CAD build for the part. Positions are in the model's coordinates, mm. A direction names the side the tool comes from. Round coordinates to 2 decimals unless told otherwise and drop trailing zeros. Order: outer loops, then holes, each group sorted by start corner. A loop starts at its lowest first (then second) coordinate and runs counter-clockwise, first axis right, second up. Notation, with made-up numbers: (69.5, 16) -> (109.5, 16) arc R7 cw to (109.5, 27) -> close; hole circle Ø10 at (-32, -38.75). An arc over 180 degrees is marked (long way). Return JSON: item names as keys, results as strings. Group by question number.
Q1. Cut at B-B (y = 12.25). Write the cut outline in (x, z), then the cut area to 3 significant figures.
Q2. Mould opens along X. For faces 1 (the flat face through (-12, 6, -11.3)), 2 (the cylindrical face through (18.521, 6.374, -3.794)), 3 (the flat face through (-20, 11, 0)) say: +X half, -X half, draft (parallel to the pull), parting line (faces both ways), or undercut.
Q3. Cut at C-C (z = -0.75). Write the cut outline in (x, y).
Q4. Probe line 1 along X through (y, z) = (7.75, -10.75); line 2 along X through (y, z) = (8.75, 9.5); line 3 along Z through (x, y) = (-10.5, 12.5). List the from-to ranges inside material, lowest first.
Q5. Flat gauge pins, fed straight in: pin 1 (2 mm diameter, centred on x = -12, z = -10.5, fed in from +Y); pin 2 (1.6 mm diameter, centred on x = -11.5, y = 6.5, fed in from -Z). Where does each tip first touch, or does it go through?
Q6. Cut at D-D (z = 2.5). Write the cut outline in (x, y), then the cut area to 3 significant figures.
Q7. Cut at A-A (x = 12.5). Write the cut outline in (y, z).
Q8. Which spindle directions (+Z, -Z, +X, -X, +Y, -Y) get a long thin tool onto all of the face, cutting with end or side? Do faces 4 (the flat face through (0, 8.5, 11)), 5 (the flat face through (19, 10, 2)), 6 (the flat face through (-17, 10, 0)). Say none if no direction does.
from build123d import *

# Parameters (mm, degrees)
SKETCH1_W            = 40
SKETCH1_H            = 24.6
SKETCH1_W_2          = 34
SKETCH1_H_2          = 18.6
BOSS_EXTRUDE1_DEPTH  = 14
CUT_EXTRUDE1_DEPTH   = 10
SKETCH5_W            = 4
SKETCH5_H            = 3
CUT_EXTRUDE2_DEPTH   = 10
BOSS_EXTRUDE2_DEPTH  = 40
BOSS_EXTRUDE3_DEPTH  = 40
SKETCH8_W            = 4
SKETCH8_H            = 12
BOSS_EXTRUDE4_DEPTH  = 1
FILLET4_R            = 21
SKETCH10_W           = 4
SKETCH10_H           = 2
BOSS_EXTRUDE6_DEPTH  = 1
SKETCH13_W           = 2
SKETCH13_H           = 3
BOSS_EXTRUDE7_DEPTH  = 1
SKETCH14_W           = 2
SKETCH14_H           = 1.5
BOSS_EXTRUDE9_DEPTH  = 1
SKETCH14_4_W         = 2
SKETCH14_4_H         = 1.5
BOSS_EXTRUDE10_DEPTH = 1
CUT_EXTRUDE5_DEPTH   = 28
CUT_EXTRUDE6_DEPTH   = 28
FILLET7_R            = 0.25
SKETCH18_W           = 34
SKETCH18_H           = 18.6
BOSS_EXTRUDE11_DEPTH = 1.25
CUT_EXTRUDE7_DEPTH   = 5.25
SKETCH20_W           = 4
SKETCH20_H           = 2
CUT_EXTRUDE8_DEPTH   = 5.25
SKETCH21_W           = 2
SKETCH21_H           = 1.5
CUT_EXTRUDE9_DEPTH   = 5.25


with BuildPart() as part:
    # Sketch1 → Boss-Extrude1 (new body)
    with BuildSketch(Plane(origin=(0, 0, 0), x_dir=(1, 0, 0), z_dir=(0, 1, 0))):
        Rectangle(SKETCH1_W, SKETCH1_H)
        Rectangle(SKETCH1_W_2, SKETCH1_H_2, mode=Mode.SUBTRACT)
    extrude(amount=BOSS_EXTRUDE1_DEPTH)

    # Sketch3 → Cut-Extrude1 (cut)
    with BuildSketch(Plane(origin=(20, 0, 0), x_dir=(0, 0, -1), z_dir=(1, 0, 0))):
        with BuildLine():
            ThreePointArc((2.9, 4.25), (4.15, 5.5), (2.9, 6.75))
            Line((2.9, 6.75), (-2.9, 6.75))
            ThreePointArc((-2.9, 6.75), (-4.15, 5.5), (-2.9, 4.25))
            Line((-2.9, 4.25), (2.9, 4.25))
        make_face()
    extrude(amount=-CUT_EXTRUDE1_DEPTH, mode=Mode.SUBTRACT)


with BuildPart() as body_2:
    # Split1: the piece on the far side of the plane
    add(part.part)
    split(bisect_by=Plane(origin=(0, 5.5, 0), x_dir=(0, 0, -1), z_dir=(0, -1, 0)), keep=Keep.BOTTOM)

    # Sketch5 → Cut-Extrude2 (cut)
    with BuildSketch(Plane(origin=(20, 0, 0), x_dir=(0, 0, -1), z_dir=(1, 0, 0))):
        with Locations((0, 9.75)):
            Rectangle(SKETCH5_W, SKETCH5_H)
    extrude(amount=-CUT_EXTRUDE2_DEPTH, mode=Mode.SUBTRACT)

    # Sketch6 → Boss-Extrude2 (add)
    with BuildSketch(Plane(origin=(20, 0, 0), x_dir=(0, 0, -1), z_dir=(1, 0, 0))):
        with BuildLine():
            Line((-9.3, 17), (9.3, 17))
            ThreePointArc((9.3, 17), (11.421320344, 16.121320344), (12.3, 14))
            Line((12.3, 14), (-12.3, 14))
            ThreePointArc((-12.3, 14), (-11.421320344, 16.121320344), (-9.3, 17))
        make_face()
    extrude(amount=-BOSS_EXTRUDE2_DEPTH)


with BuildPart() as part_1:
    add(part.part)

    # Split1
    split(bisect_by=Plane(origin=(0, 5.5, 0), x_dir=(0, 0, -1), z_dir=(0, -1, 0)), keep=Keep.TOP)

    # Sketch7 → Boss-Extrude3 (add)
    with BuildSketch(Plane.ZY.offset(20)):
        with BuildLine():
            Line((-9.3, -3), (9.3, -3))
            ThreePointArc((9.3, -3), (11.421320344, -2.121320344), (12.3, 0))
            Line((12.3, 0), (-12.3, 0))
            ThreePointArc((-12.3, 0), (-11.421320344, -2.121320344), (-9.3, -3))
        make_face()
    extrude(amount=-BOSS_EXTRUDE3_DEPTH)

    # Sketch8 → Boss-Extrude4 (add)
    with BuildSketch(Plane.XY.offset(12.3)):
        with Locations((0, 6.5)):
            Rectangle(SKETCH8_W, SKETCH8_H)
    extrude(amount=BOSS_EXTRUDE4_DEPTH)

    # Fillet4
    # the kernel refuses this fillet: 21 mm, written as the material it takes off along each edge
    with BuildSketch(Plane(origin=(18.007810594, 0.5, 13.3), x_dir=(0, 0, -1), z_dir=(-1, 0, 0))) as fillet4_piece_1:
        with BuildLine():
            CenterArc((21, -6.403124237), FILLET4_R, 162.247209838, 17.752790162)
            Line((0, -6.403124237), (-0.42, -6.403124237))
            Line((-0.42, -6.403124237), (-0.42, 0))
            Line((-0.42, 0), (0, 0.42))
            ThreePointArc((0, 0.42), (0.5, 0.42), (0.6, 0.128062485))
            Line((0.6, 0.128062485), (1, 0))
        make_face()
    extrude(amount=36.015621187, mode=Mode.SUBTRACT)

    # Sketch10 → Boss-Extrude6 (add)
    with BuildSketch(Plane(origin=(0, 0, 12.3), x_dir=(-1, 0, 0), z_dir=(0, 0, -1))):
        with Locations((0, 9.5)):
            Rectangle(SKETCH10_W, SKETCH10_H)
    extrude(amount=BOSS_EXTRUDE6_DEPTH)

    # Sketch13 → Boss-Extrude7 (add)
    with BuildSketch(Plane(origin=(0, 0, -12.3), x_dir=(-1, 0, 0), z_dir=(0, 0, -1))):
        with Locations((-12, 7)):
            Rectangle(SKETCH13_W, SKETCH13_H)
        with Locations((12, 7)):
            Rectangle(SKETCH13_W, SKETCH13_H)
    extrude(amount=-BOSS_EXTRUDE7_DEPTH)

    # Sketch14 → Boss-Extrude9 (add)
    with BuildSketch(Plane.XY.offset(-11.3)):
        with Locations((12, 7.75)):
            Rectangle(SKETCH14_W, SKETCH14_H)
    extrude(amount=BOSS_EXTRUDE9_DEPTH)

    # Sketch14<4> → Boss-Extrude10 (add)
    with BuildSketch(Plane.XY.offset(-11.3)):
        with Locations((-12, 7.75)):
            Rectangle(SKETCH14_4_W, SKETCH14_4_H)
        with Locations((12, 7.75)):
            Rectangle(SKETCH14_4_W, SKETCH14_4_H)
    extrude(amount=BOSS_EXTRUDE10_DEPTH)

    # Sketch15 → Cut-Extrude5 (cut)
    with BuildSketch(Plane(origin=(13, 0, 0), x_dir=(0, 0, -1), z_dir=(1, 0, 0))):
        Polygon((10.3, 7), (11.3, 8.5), (10.3, 8.5), align=None)
    extrude(amount=-CUT_EXTRUDE5_DEPTH, mode=Mode.SUBTRACT)

    # Sketch16 → Cut-Extrude6 (cut)
    with BuildSketch(Plane(origin=(2, 0, 0), x_dir=(0, 0, -1), z_dir=(1, 0, 0))):
        Polygon((-13.3, 12.5), (-12.3, 10.5), (-12.3, 12.5), align=None)
    extrude(amount=-CUT_EXTRUDE6_DEPTH, mode=Mode.SUBTRACT)

    # Fillet7
    fillet7_edges = [part_1.edges().sort_by_distance(p)[0] for p in [
        (0, 12.5, 13.3),
    ]]
    fillet(fillet7_edges, radius=FILLET7_R)

    # Sketch18 → Boss-Extrude11 (add)
    with BuildSketch(Plane(origin=(0, 0, 0), x_dir=(1, 0, 0), z_dir=(0, 1, 0))):
        Rectangle(SKETCH18_W, SKETCH18_H)
    extrude(amount=BOSS_EXTRUDE11_DEPTH)

    # Sketch19 → Cut-Extrude7 (cut)
    with BuildSketch(Plane.ZY.offset(2)):
        Polygon((12.3, 10.5), (11.3, 8.5), (11.3, 10.5), align=None)
    extrude(amount=-CUT_EXTRUDE7_DEPTH, mode=Mode.SUBTRACT)


with BuildPart() as body_2_1:
    add(body_2.part)

    # Combine3: cut part
    add(part_1.part, mode=Mode.SUBTRACT)

    # Sketch20 → Cut-Extrude8 (cut)
    with BuildSketch(Plane.XY.offset(12.3)):
        with Locations((0, 9.5)):
            Rectangle(SKETCH20_W, SKETCH20_H)
    extrude(amount=-CUT_EXTRUDE8_DEPTH, mode=Mode.SUBTRACT)

    # Sketch21 → Cut-Extrude9 (cut)
    with BuildSketch(Plane(origin=(0, 0, -12.3), x_dir=(-1, 0, 0), z_dir=(0, 0, -1))):
        with Locations((-12, 7.75)):
            Rectangle(SKETCH21_W, SKETCH21_H)
        with Locations((12, 7.75)):
            Rectangle(SKETCH21_W, SKETCH21_H)
    extrude(amount=-CUT_EXTRUDE9_DEPTH, mode=Mode.SUBTRACT)


solid = body_2_1.part
Solution:
{
 "1": {"outline": "(-20, -12.3) -> (20, -12.3) -> (20, 12.3) -> (-20, 12.3) -> close; hole (-17, -9.3) -> (17, -9.3) -> (17, 9.3) -> (-17, 9.3) -> close", "area": "352 mm²"},
 "2": {"face 1": "undercut", "face 2": "draft", "face 3": "-X half"},
 "3": {"outline": "(-20, 5.5) -> (-17, 5.5) -> (-17, 14) -> (17, 14) -> (17, 11.25) -> (20, 11.25) -> (20, 17) -> (-20, 17) -> close; (17, 6.75) -> (20, 6.75) -> (20, 8.25) -> (17, 8.25) -> close"},
 "4": {"line 1": "x = -20 to -13, -11 to 11, 13 to 20", "line 2": "x = -20 to -2, 2 to 20", "line 3": "z = -12.3 to -9.3, 9.3 to 12.3"},
 "5": {"pin 1": "stops at y = 16.99", "pin 2": "stops at z = -12.3"},
 "6": {"outline": "(-20, 5.5) -> (-17, 5.5) -> (-17, 14) -> (17, 14) -> (17, 6.75) -> (20, 6.75) -> (20, 17) -> (-20, 17) -> close", "area": "167 mm²"},
 "7": {"outline": "(5.5, -11.3) -> (7, -11.3) -> (7, -9.3) -> (5.5, -9.3) -> close; (5.5, 9.3) -> (14, 9.3) -> (14, -9.3) -> (8.5, -9.3) -> (8.5, -12.3) -> (14, -12.3) arc R3 ccw to (17, -9.3) -> (17, 9.3) arc R3 ccw to (14, 12.3) -> (5.5, 12.3) -> close"},
 "8": {"face 4": "+Z", "face 5": "+X", "face 6": "-Y"}
}
